Input: part model. Units: mm. Frame: model coordinates. Coordinates: 2 decimals unless noted, no trailing zeros. Write each loop counter-clockwise with the first axis right and the second up, starting at its lowest first coordinate (ties: lowest second). Pieces come first, ordered by that corner, then holes. Notation, with made-up numbers: (-5, -9) - (32, -9) arc R10 ccw to (32, -5) - close; hole circle Ø11 at (82.5, 11.5). An arc over 180 degrees is marked (long way). One line per question, with ' | ' between items. Start each with the question number.
1) Line query: line 1 (X direction, y = 5.5, z = -9); line 2 (Y direction, x = 224, z = -8.75); line 3 (Y direction, x = 220.5, z = -4.25). Output: solid intervals per line, ascending.
2) First-contact query: P1, Ø5, axis at x = 156, z = -2.5, coming from the +Y side; P2, Ø2, axis at x = 166.5, z = -1, coming from the +Y side; P3, Ø2, axis at x = 50.5, y = 6.5, coming from the -Z side. Flat tips, straight axial feed; report the tip coordinate or a pass-through.
3) Section query A-A on x = 216. Return loops of the section in (y, z), and give its area (3 significant figures).
4) Section query B-B on z = -1.5. Return loops of the section in (x, y).
```python
from build123d import *

# Parameters (mm, degrees)
SKETCH2_W           = 250
SKETCH2_H           = 10
BOSS_EXTRUDE1_DEPTH = 3
SKETCH3_W           = 5
SKETCH3_H           = 10
BOSS_EXTRUDE2_DEPTH = 8
BOSS_EXTRUDE3_REACH = 247
SKETCH4_R           = 0.75
SKETCH5_W           = 16.35970525
SKETCH5_H           = 10
BOSS_EXTRUDE4_DEPTH = 8
SKETCH6_R           = 1.4956439
SKETCH6_R_2         = 1.153364649
BOSS_EXTRUDE5_DEPTH = 8


with BuildPart() as part:
    # Sketch2 → Boss-Extrude1 (new body)
    with BuildSketch(Plane(origin=(0, 0, 0), x_dir=(1, 0, 0), z_dir=(0, 1, 0))):
        with Locations((125, 5)):
            Rectangle(SKETCH2_W, SKETCH2_H)
    extrude(amount=BOSS_EXTRUDE1_DEPTH)

    # Sketch3 → Boss-Extrude2 (add)
    with BuildSketch(Plane(origin=(0, 3, 0), x_dir=(1, 0, 0), z_dir=(0, 1, 0))):
        with Locations((2.5, 5)):
            Rectangle(SKETCH3_W, SKETCH3_H)
        with Locations((247.5, 5)):
            Rectangle(SKETCH3_W, SKETCH3_H)
    extrude(amount=BOSS_EXTRUDE2_DEPTH)

    # Sketch4 → Boss-Extrude3 (add, up to next)
    with BuildSketch(Plane(origin=(5, 0, 0), x_dir=(0, 0, -1), z_dir=(1, 0, 0)), mode=Mode.PRIVATE) as boss_extrude3_sk1:
        with Locations((4.754905599, 7.100772806)):
            Circle(SKETCH4_R)
    boss_extrude3_tool1 = extrude(boss_extrude3_sk1.sketch, amount=BOSS_EXTRUDE3_REACH, mode=Mode.PRIVATE) - part.part
    add(boss_extrude3_tool1.solids().sort_by_distance((5, 7.100773, -4.754906))[0])

    # Sketch5 → Boss-Extrude4 (add)
    with BuildSketch(Plane(origin=(0, 3, 0), x_dir=(1, 0, 0), z_dir=(0, 1, 0))):
        with Locations((22.45057465, 5)):
            Rectangle(SKETCH5_W, SKETCH5_H)
    extrude(amount=BOSS_EXTRUDE4_DEPTH)

    # Sketch6 → Boss-Extrude5 (add)
    with BuildSketch(Plane.ZY.offset(-14.270722025)):
        with Locations((-4.800860799, 7.162046407)):
            Circle(SKETCH6_R)
        with Locations((-4.800860799, 7.162046407)):
            Circle(SKETCH6_R_2, mode=Mode.SUBTRACT)
    extrude(amount=BOSS_EXTRUDE5_DEPTH)


solid = part.part
```
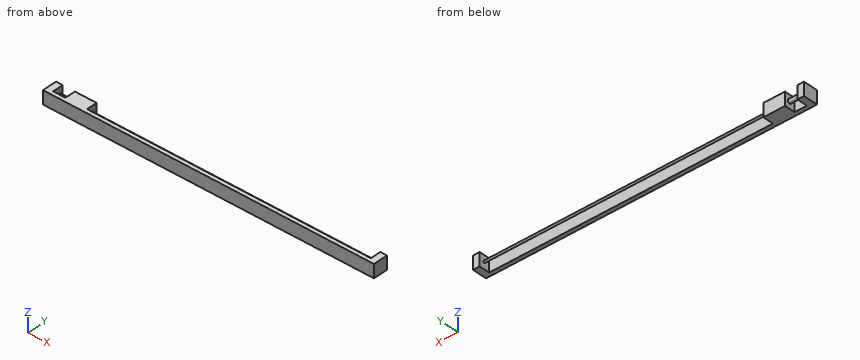
Answer key:
1) line 1: 0 to 5, 14.27 to 30.63, 245 to 250 | line 2: 0 to 3 | line 3: 0 to 3, 6.55 to 7.66
2) P1: y = 7.85 | P2: y = 3 | P3: z = -5.5
3) outline: (0, -10) - (3, -10) - (3, 0) - (0, 0) - close; circle Ø1.5 at (7.1, -4.75) | area: 31.8 mm²
4) outline: (0, 0) - (250, 0) - (250, 11) - (245, 11) - (245, 3) - (30.63, 3) - (30.63, 11) - (14.27, 11) - (14.27, 3) - (5, 3) - (5, 11) - (0, 11) - close
